from build123d import *

# Parameters (mm, degrees)
P_IDAT_VYSUNUT_M1_DEPTH = 3


with BuildPart() as part:
    # Skica1 → Přidat vysunutím1 (new body)
    with BuildSketch(Plane.XY):
        Polygon((0, 3), (15, 3), (15, 0), (32.38, 0), (32.38, 3), (47.38, 3), (47.38, 59), (32.38, 59), (32.38, 62), (15, 62), (15, 59), (0, 59), align=None)
        Polygon((12.227967454, 31), (12.227967454, 45.5), (15.539999999, 45.5), (15.539999999, 47), (31.839999999, 47), (31.839999999, 45.5), (35.152032457, 45.5), (35.152032457, 31), (35.152032457, 20), (32.652032457, 20), (32.652032457, 8.6), (14.727967454, 8.6), (14.727967454, 20), (12.227967454, 20), align=None, mode=Mode.SUBTRACT)
    extrude(amount=P_IDAT_VYSUNUT_M1_DEPTH)


solid = part.part
Design review of the part built by this model. Coordinates are the model's own, in mm. A direction names the side the tool comes from. Round coordinates to 2 decimals unless told otherwise and drop trailing zeros. Order: outer loops, then holes, each group sorted by start corner. A loop starts at its lowest first (then second) coordinate and runs counter-clockwise, first axis right, second up. Notation, with made-up numbers: M 16,1 L 55,1 A16 ccw 55,19 Z; hole C -31.75,26.25 d7. An arc over 180 degrees is marked long. Answer as CSV lines item,"result". Start each with the question number.
1) Add section D-D (x = 42.5). Give the boundary of the cut face in (y, z).
2) For pin 1 Ø0.9 at (y, z) = (61, 1) entering from +X; pin 2 Ø1.5 at (x, z) = (7, 1) entering from -Y, all flat-tipped, find the tip position at first contact; note any pin that passes through.
3) Add section A-A (x = 17.5). Give the boundary of the cut face in (y, z).
4) Add section C-C (z = 1.3). Give the boundary of the cut face in (x, y).
5) The part is to be moulded in two halves that separate along X. For faces 1 (the face through (8, 31, 3)), 2 (the face through (24, 8.6, 1)), 3 (the face through (47.38, 31, 1)), say which applies: +X half, -X half, draft (parallel to the pull), parting line (faces both ways), or undercut.
6) Tool access review of faces 4 (the face through (15, 2, 1)), 5 (the face through (32.38, 1, 1)), 6 (the face through (31.84, 46, 1)), 7 (the face through (40, 59, 1)): name each direction out of +Z, -Z, +X, -X, +Y, -Y from which nothing blocks a thin tool from reaching the whole face with its end or side.
7) Add section B-B (y = 14.5). Give the boundary of the cut face in (x, z), then the cut area to 3 significant figures.
8) Wall thickness on line 1 along X through (y, z) = (44, 2.05); line 2 along Y through (x, z) = (33.5, 2.3); line 3 along Y through (x, z) = (22.5, 0.6): over which ranges is each line inside the solid? List them lowest first. Write a range as [from, to].
Resolved:
1,outline,"M 3,0 L 59,0 L 59,3 L 3,3 Z"
2,pin 1,"x = 32.38"
2,pin 2,"y = 3"
3,outline,"M 0,0 L 8.6,0 L 8.6,3 L 0,3 Z; M 47,0 L 62,0 L 62,3 L 47,3 Z"
4,outline,"M 0,3 L 15,3 L 15,0 L 32.38,0 L 32.38,3 L 47.38,3 L 47.38,59 L 32.38,59 L 32.38,62 L 15,62 L 15,59 L 0,59 Z; hole M 12.23,20 L 14.73,20 L 14.73,8.6 L 32.65,8.6 L 32.65,20 L 35.15,20 L 35.15,45.5 L 31.84,45.5 L 31.84,47 L 15.54,47 L 15.54,45.5 L 12.23,45.5 Z"
5,face 1,"draft"
5,face 2,"undercut"
5,face 3,"+X half"
6,face 4,"+Z, -Z, -X, -Y"
6,face 5,"+Z, -Z, +X, -Y"
6,face 6,"+Z, -Z"
6,face 7,"+Z, -Z, +X, +Y"
7,outline,"M 0,0 L 14.73,0 L 14.73,3 L 0,3 Z; M 32.65,0 L 47.38,0 L 47.38,3 L 32.65,3 Z"
7,area,"88.4 mm^2"
8,line 1,"[0, 12.23], [35.15, 47.38]"
8,line 2,"[3, 20], [45.5, 59]"
8,line 3,"[0, 8.6], [47, 62]"
